Build history of the part. All positions in model axes, mm. Face numbers are marked on the shaded views. Round coordinates to 2 decimals unless told otherwise and drop trailing zeros. Write each loop counter-clockwise with the first axis right and the second up, starting at its lowest first coordinate (ties: lowest second). Pieces come first, ordered by that corner, then holes.
Item 1: Band-saw the part on B-B, the plane x = 0. Write the cut outline in (y, z).
Item 2: Band-saw the part on D-D, the plane z = 7.25. Write the cut outline in (x, y), then the cut area to 3 significant figures.
Item 3: Band-saw the part on C-C, the plane y = 18. Write the cut outline in (x, z).
Item 4: Mould opens along Y. For the marked faces 1 and 2 say: +Y half, -Y half, draft (parallel to the pull), parting line (faces both ways), or undercut.
Item 5: Band-saw the part on A-A, the plane x = 17.5. Write the cut outline in (y, z), then the cut area to 3 significant figures.
Item 6: Drop flat-ended pins along their axis: pin 1 Ø2 at (x, y) = (-14.56, 25.22) entering from +Z; pin 2 Ø3 at (x, y) = (-14.56, -25.22) entering from +Z; pin 3 Ø6 at (x, y) = (-35, 0) entering from +Z; pin 4 Ø1 at (y, z) = (6, 1) entering from -X. Give the stop position or say it passes through.
Item 7: Wall check: probe 1 along Y at (x, z) = (17.5, 0.6); probe 2 along Y at (x, z) = (0, 2.1); probe 3 along Z at (x, y) = (-4.5, 21). Give the ranges that are in metal, low to high.
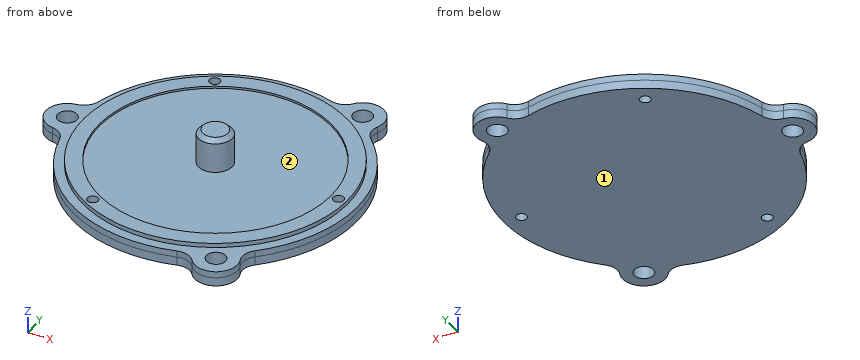
```python
from build123d import *

# Parameters (mm, degrees)
ESQUISSE1_R                        = 31.25
BOSS_EXTRU_1_DEPTH                 = 2
BOSS_EXTRU_2_DEPTH                 = 25.5
BOSS_EXTRU_2_DEPTH_BACK            = 2
ESQUISSE2_R                        = 33.25
ESQUISSE2_R_2                      = 31.25
ESQUISSE3_R                        = 7.95
BOSS_EXTRU_3_DEPTH                 = 7.5
ESQUISSE4_R                        = 3.95
BOSS_EXTRU_4_DEPTH                 = 8
CHANFREIN1_SIZE                    = 1
BOSS_EXTRU_5_DEPTH                 = 27.5
ESQUISSE6_R                        = 1.75
ENL_V_MAT_EXTRU_1_DEPTH            = 10
CONG_1_R                           = 4
R_P_TITION_CIRCULAIRE2_COUNT       = 3
CONG_1_OF_R_P_TITION_CIRCULAIRE2_R = 4
ENL_V_MAT_EXTRU_2_DEPTH            = 25.5
ESQUISSE8_R                        = 3.95
BOSS_EXTRU_6_DEPTH                 = 8
ESQUISSE9_R                        = 2.25
ENL_V_MAT_EXTRU_3_DEPTH            = 54.952376281
CHANFREIN2_SIZE                    = 1
ESQUISSE10_R                       = 31
ESQUISSE10_R_2                     = 27.25
BOSS_EXTRU_7_DEPTH                 = 0.5
ESQUISSE11_R                       = 31
ENL_V_MAT_EXTRU_4_DEPTH            = 0.5
ESQUISSE12_R                       = 2.25
BOSS_EXTRU_8_DEPTH                 = 2
ESQUISSE13_R                       = 1.25
ENL_V_MAT_EXTRU_5_DEPTH            = 54.88050581


with BuildPart() as part:
    # Esquisse1 → Boss.-Extru.1 (new body)
    with BuildSketch(Plane.XY):
        Circle(ESQUISSE1_R)
    extrude(amount=BOSS_EXTRU_1_DEPTH)

    # Esquisse2 → Boss.-Extru.2 (add, two sides: drawn at the far end of the back side and taken through both)
    with BuildSketch(Plane.XY.offset(2).offset(-BOSS_EXTRU_2_DEPTH_BACK)):
        Circle(ESQUISSE2_R)
        Circle(ESQUISSE2_R_2, mode=Mode.SUBTRACT)
    extrude(amount=BOSS_EXTRU_2_DEPTH + BOSS_EXTRU_2_DEPTH_BACK)

    # Esquisse3 → Boss.-Extru.3 (add)
    with BuildSketch(Plane.XY.offset(2)):
        Circle(ESQUISSE3_R)
    extrude(amount=BOSS_EXTRU_3_DEPTH)

    # Esquisse4 → Boss.-Extru.4 (add)
    with BuildSketch(Plane.XY.offset(9.5)):
        Circle(ESQUISSE4_R)
    extrude(amount=BOSS_EXTRU_4_DEPTH)

    # Chanfrein1
    chanfrein1_edges = [part.edges().sort_by_distance(p)[0] for p in [
        (-7.95, 0, 9.5),
        (-3.95, 0, 17.5),
    ]]
    chamfer(chanfrein1_edges, length=CHANFREIN1_SIZE)

    # Esquisse5 → Boss.-Extru.5 (add)
    with BuildSketch(Plane.XY.offset(27.5)):
        with BuildLine():
            ThreePointArc((-32.936607143, -4.554383594), (-40, 0), (-32.936607143, 4.554383594))
            ThreePointArc((-32.936607143, 4.554383594), (-33.25, 0), (-32.936607143, -4.554383594))
        make_face()
    boss_extru_5 = extrude(amount=-BOSS_EXTRU_5_DEPTH)

    # Esquisse6 → Enlèv. mat.-Extru.1 (cut)
    with BuildSketch(Plane.XY.offset(27.5)):
        with Locations((-35, 0)):
            Circle(ESQUISSE6_R)
    enl_v_mat_extru_1 = extrude(amount=-ENL_V_MAT_EXTRU_1_DEPTH, mode=Mode.SUBTRACT)

    # Congé1
    cong_1_edges = [part.edges().sort_by_distance(p)[0] for p in [
        (-32.936607143, 4.554383594, 13.75),
        (-32.936607143, -4.554383594, 13.75),
    ]]
    fillet(cong_1_edges, radius=CONG_1_R)

    # Répétition circulaire2: Boss.-Extru.5, Enlèv. mat.-Extru.1 ×3 about axis
    r_p_tition_circulaire2_axis = Axis((0, 0, 0), (0, 0, 1))
    add([boss_extru_5.rotate(r_p_tition_circulaire2_axis, i * 360 / R_P_TITION_CIRCULAIRE2_COUNT) for i in range(1, R_P_TITION_CIRCULAIRE2_COUNT)])
    add([enl_v_mat_extru_1.rotate(r_p_tition_circulaire2_axis, i * 360 / R_P_TITION_CIRCULAIRE2_COUNT) for i in range(1, R_P_TITION_CIRCULAIRE2_COUNT)], mode=Mode.SUBTRACT)

    # Congé1 of Répétition circulaire2
    cong_1_of_r_p_tition_circulaire2_edges = [part.edges().sort_by_distance(p)[0] for p in [
        (12.524091681, -30.801130297, 13.75),
        (20.412515462, -26.246746703, 13.75),
        (20.412515462, 26.246746703, 13.75),
        (12.524091681, 30.801130297, 13.75),
    ]]
    fillet(cong_1_of_r_p_tition_circulaire2_edges, radius=CONG_1_OF_R_P_TITION_CIRCULAIRE2_R)

    # Esquisse7 → Enlèv. mat.-Extru.2 (cut)
    with BuildSketch(Plane.XY.offset(27.5)):
        with BuildLine():
            ThreePointArc((-35.647321429, 4.957920428), (-40, 0), (-35.647321429, -4.957920428))
            ThreePointArc((-35.647321429, -4.957920428), (-33.49964623, -5.941818617), (-32.281669463, -7.965947318))
            ThreePointArc((-32.281669463, -7.965947318), (-16.625, -28.795344676), (9.242121989, -31.939719491))
            ThreePointArc((9.242121989, -31.939719491), (11.604057248, -31.982453961), (13.529975674, -33.350446148))
            ThreePointArc((13.529975674, -33.350446148), (20, -34.641016151), (22.117345755, -28.39252572))
            ThreePointArc((22.117345755, -28.39252572), (21.895588982, -26.040635345), (23.039547474, -23.973772173))
            ThreePointArc((23.039547474, -23.973772173), (33.25, 0), (23.039547474, 23.973772173))
            ThreePointArc((23.039547474, 23.973772173), (21.895588982, 26.040635345), (22.117345755, 28.39252572))
            ThreePointArc((22.117345755, 28.39252572), (20, 34.641016151), (13.529975674, 33.350446148))
            ThreePointArc((13.529975674, 33.350446148), (11.604057248, 31.982453961), (9.242121989, 31.939719491))
            ThreePointArc((9.242121989, 31.939719491), (-16.625, 28.795344676), (-32.281669463, 7.965947318))
            ThreePointArc((-32.281669463, 7.965947318), (-33.49964623, 5.941818617), (-35.647321429, 4.957920428))
        make_face()
    extrude(amount=-ENL_V_MAT_EXTRU_2_DEPTH, mode=Mode.SUBTRACT)

    # Esquisse8 → Boss.-Extru.6 (add)
    with BuildSketch(Plane.XY.offset(2)):
        Circle(ESQUISSE8_R)
    extrude(amount=BOSS_EXTRU_6_DEPTH)

    # Esquisse9 → Enlèv. mat.-Extru.3 (cut, through all)
    with BuildSketch(Plane.XY.offset(2)):
        with Locations((-35, 0)):
            Circle(ESQUISSE9_R)
        with Locations((17.5, 30.310889132)):
            Circle(ESQUISSE9_R)
        with Locations((17.5, -30.310889132)):
            Circle(ESQUISSE9_R)
    extrude(amount=-ENL_V_MAT_EXTRU_3_DEPTH, mode=Mode.SUBTRACT)

    # Chanfrein2
    chanfrein2_edges = [part.edges().sort_by_distance(p)[0] for p in [
        (-3.95, 0, 10),
    ]]
    chamfer(chanfrein2_edges, length=CHANFREIN2_SIZE)

    # Esquisse10 → Boss.-Extru.7 (add)
    with BuildSketch(Plane.XY.offset(2)):
        Circle(ESQUISSE10_R)
        Circle(ESQUISSE10_R_2, mode=Mode.SUBTRACT)
    extrude(amount=BOSS_EXTRU_7_DEPTH)

    # Esquisse11 → Enlèv. mat.-Extru.4 (cut)
    with BuildSketch(Plane.XY.offset(2)):
        with BuildLine():
            ThreePointArc((-35.647321429, 4.957920428), (-33.49964623, 5.941818617), (-32.281669463, 7.965947318))
            ThreePointArc((-32.281669463, 7.965947318), (-16.625, 28.795344676), (9.242121989, 31.939719491))
            ThreePointArc((9.242121989, 31.939719491), (11.604057248, 31.982453961), (13.529975674, 33.350446148))
            ThreePointArc((13.529975674, 33.350446148), (20, 34.641016151), (22.117345755, 28.39252572))
            ThreePointArc((22.117345755, 28.39252572), (21.895588982, 26.040635345), (23.039547474, 23.973772173))
            ThreePointArc((23.039547474, 23.973772173), (33.25, 0), (23.039547474, -23.973772173))
            ThreePointArc((23.039547474, -23.973772173), (21.895588982, -26.040635345), (22.117345755, -28.39252572))
            ThreePointArc((22.117345755, -28.39252572), (20, -34.641016151), (13.529975674, -33.350446148))
            ThreePointArc((13.529975674, -33.350446148), (11.604057248, -31.982453961), (9.242121989, -31.939719491))
            ThreePointArc((9.242121989, -31.939719491), (-16.625, -28.795344676), (-32.281669463, -7.965947318))
            ThreePointArc((-32.281669463, -7.965947318), (-33.49964623, -5.941818617), (-35.647321429, -4.957920428))
            ThreePointArc((-35.647321429, -4.957920428), (-40, 0), (-35.647321429, 4.957920428))
        make_face()
        Circle(ESQUISSE11_R, mode=Mode.SUBTRACT)
    extrude(amount=-ENL_V_MAT_EXTRU_4_DEPTH, mode=Mode.SUBTRACT)

    # Esquisse12 → Boss.-Extru.8 (add)
    with BuildSketch(Plane(origin=(0, 0, 0), x_dir=(-1, 0, 0), z_dir=(0, 0, -1))):
        with BuildLine():
            ThreePointArc((35.647321429, -4.957920428), (40, 0), (35.647321429, 4.957920428))
            ThreePointArc((35.647321429, 4.957920428), (33.49964623, 5.941818617), (32.281669463, 7.965947318))
            ThreePointArc((32.281669463, 7.965947318), (16.625, 28.795344676), (-9.242121989, 31.939719491))
            ThreePointArc((-9.242121989, 31.939719491), (-11.604057248, 31.982453961), (-13.529975674, 33.350446148))
            ThreePointArc((-13.529975674, 33.350446148), (-20, 34.641016151), (-22.117345755, 28.39252572))
            ThreePointArc((-22.117345755, 28.39252572), (-21.895588982, 26.040635345), (-23.039547474, 23.973772173))
            ThreePointArc((-23.039547474, 23.973772173), (-33.25, 0), (-23.039547474, -23.973772173))
            ThreePointArc((-23.039547474, -23.973772173), (-21.895588982, -26.040635345), (-22.117345755, -28.39252572))
            ThreePointArc((-22.117345755, -28.39252572), (-20, -34.641016151), (-13.529975674, -33.350446148))
            ThreePointArc((-13.529975674, -33.350446148), (-11.604057248, -31.982453961), (-9.242121989, -31.939719491))
            ThreePointArc((-9.242121989, -31.939719491), (16.625, -28.795344676), (32.281669463, -7.965947318))
            ThreePointArc((32.281669463, -7.965947318), (33.49964623, -5.941818617), (35.647321429, -4.957920428))
        make_face()
        with Locations(Location((35, 0, 0), (0, 0, 180))):
            Circle(ESQUISSE12_R, mode=Mode.SUBTRACT)
        with Locations(Location((-17.5, -30.310889132, 0), (0, 0, 180))):
            Circle(ESQUISSE12_R, mode=Mode.SUBTRACT)
        with Locations(Location((-17.5, 30.310889132, 0), (0, 0, 180))):
            Circle(ESQUISSE12_R, mode=Mode.SUBTRACT)
    extrude(amount=BOSS_EXTRU_8_DEPTH)

    # Esquisse13 → Enlèv. mat.-Extru.5 (cut, through all)
    with BuildSketch(Plane.XY.offset(2.5)):
        with Locations((-14.5625, 25.222989885)):
            Circle(ESQUISSE13_R)
        with Locations((29.125, 0)):
            Circle(ESQUISSE13_R)
        with Locations((-14.5625, -25.222989885)):
            Circle(ESQUISSE13_R)
    extrude(amount=-ENL_V_MAT_EXTRU_5_DEPTH, mode=Mode.SUBTRACT)


solid = part.part
```
Results:
1. outline: (-33.25, -2) - (33.25, -2) - (33.25, 1.5) - (31, 1.5) - (31, 2.5) - (27.25, 2.5) - (27.25, 2) - (3.95, 2) - (3.95, 9) - (2.95, 10) - (-2.95, 10) - (-3.95, 9) - (-3.95, 2) - (-27.25, 2) - (-27.25, 2.5) - (-31, 2.5) - (-31, 1.5) - (-33.25, 1.5) - close
2. outline: circle Ø7.9 at (0, 0)
2. area: 49.0 mm2
3. outline: (-27.96, -2) - (27.96, -2) - (27.96, 1.5) - (25.24, 1.5) - (25.24, 2.5) - (20.46, 2.5) - (20.46, 2) - (-20.46, 2) - (-20.46, 2.5) - (-25.24, 2.5) - (-25.24, 1.5) - (-27.96, 1.5) - close
4. face 1: draft
4. face 2: undercut
5. outline: (-35.31, -2) - (-32.56, -2) - (-32.56, 1.5) - (-35.31, 1.5) - close; (-28.06, -2) - (28.06, -2) - (28.06, 1.5) - (25.59, 1.5) - (25.59, 2.5) - (20.89, 2.5) - (20.89, 2) - (-20.89, 2) - (-20.89, 2.5) - (-25.59, 2.5) - (-25.59, 1.5) - (-28.06, 1.5) - close; (32.56, -2) - (35.31, -2) - (35.31, 1.5) - (32.56, 1.5) - close
5. area: 246 mm2
6. pin 1: passes through
6. pin 2: stops at z = 2.5
6. pin 3: stops at z = 1.5
6. pin 4: stops at x = -34.1
7. probe 1: y = -35.31 to -32.56, -28.06 to 28.06, 32.56 to 35.31
7. probe 2: y = -31 to -27.25, -3.95 to 3.95, 27.25 to 31
7. probe 3: z = -2 to 2
